Here's how the part is built. I have some questions about the finished solid (model axes, mm). Give positions to 0.01 mm unless a question says otherwise; leave off trailing zeros. Loops run counter-clockwise (first coordinate to the right, second up) from the corner with the lowest first, then second, coordinate; pieces in that order, holes last.
Q1. I need wall thicknesses on line 1 (Y direction, x = 0, z = 1.45); line 2 (X direction, y = 2, z = -1.2); line 3 (Y direction, x = -1.25, z = -0.9). Which ranges of each line are inside material? Lowest first, please.
Q2. If we section it at C-C (y = 15.5): Please give me the cut outline in (x, z).
Q3. If we section it at B-B (z = 1.3): Please give me the cut outline in (x, y).
Q4. If we section it at A-A (x = 0): Please give me the cut outline in (y, z), plus the area to 3 significant figures.
Q5. Will these pins go through, and if not, where does the flat tip stop? P1, Ø1.5, axis at y = 11.5, z = -1.5, coming from the -X side; P2, Ø1, axis at x = 6.5, z = -0.5, coming from the -Y side; P3, Ø1.5, axis at y = 14.5, z = -0.5, coming from the -X side.
from build123d import *


with BuildPart() as f1:
    # F0 (on Right) → F1 (revolve)
    with BuildSketch(Plane.YZ):
        with BuildLine():
            Line((-2.731482, 1.75), (-2.731482, 0))
            Line((-2.731482, 0), (-2.731482, -1.75))
            Line((-2.731482, -1.75), (-1.231482, -1.75))
            Line((-1.231482, -1.75), (-1.231482, -1))
            ThreePointArc((-1.231482, -1), (-0.524375, -0.707107), (-0.231482, 0))
            ThreePointArc((-0.231482, 0), (-0.524375, 0.707107), (-1.231482, 1))
            Line((-1.231482, 1), (-1.231482, 1.75))
            Line((-1.231482, 1.75), (-2.731482, 1.75))
        make_face()
    revolve(axis=Axis((0, 7.018518, 0.16714), (0, 0, -1)))


solid = f1.part
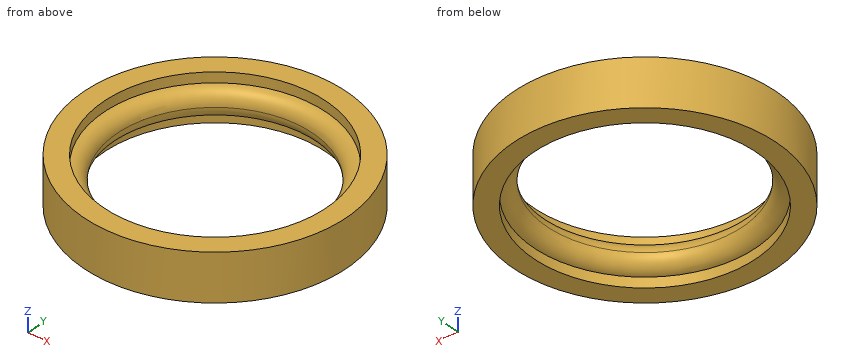
Check sheet entries:
1. line 1: y = -2.73 to -1.23, 15.27 to 16.77
1. line 2: x = -8.36 to -6.55, 6.55 to 8.36
1. line 3: y = -2.65 to -0.69, 14.73 to 16.69
2. outline: (-4.81, -1.75) - (4.81, -1.75) - (4.81, 1.75) - (-4.81, 1.75) - close
3. outline: circle Ø19.5 at (0, 7.02); hole circle Ø16.5 at (0, 7.02)
4. outline: (-2.73, -1.75) - (-1.23, -1.75) - (-1.23, -1) arc R1 ccw to (-0.23, 0) arc R1 ccw to (-1.23, 1) - (-1.23, 1.75) - (-2.73, 1.75) - close; (14.27, 0) arc R1 ccw to (15.27, -1) - (15.27, -1.75) - (16.77, -1.75) - (16.77, 1.75) - (15.27, 1.75) - (15.27, 1) arc R1 ccw to start
4. area: 13.6 mm2
5. P1: stops at x = -9.01
5. P2: stops at y = -0.67
5. P3: stops at x = -7.05
